Input: part model. Units: mm. Frame: model coordinates. A direction names the side the tool comes from. Coordinates: 2 decimals unless noted, no trailing zeros. Loops run counter-clockwise (first coordinate to the right, second up) from the corner with the lowest first, then second, coordinate; pieces in that order, holes last.
Item 1: Section A-A on z = 0. Return loops of the section in (x, y), and give its area (3 significant figures).
Item 2: Contact query for flat-ended pins moving along their axis: P1, Ø2, axis at x = -17, y = 4.5, coming from the +Z side; P2, Ø4.5, axis at x = -0.5, z = 0, coming from the +Y side; P3, Ø5.5, axis at x = -2, z = -1, coming from the -Y side. Output: stop coordinate, or through.
Item 3: Section B-B on x = -0.5. Return loops of the section in (y, z).
Item 4: Ray query, line 1 along Z through (x, y) = (-0.5, 10.45); line 2 along X through (y, z) = (-6, -22.5); line 3 along X through (y, z) = (5.5, 13). Return the intervals inside material, ascending.
Item 5: Reachability of faces 1 (the cylindrical face through (-2.25, 8.58, 0.08)), 2 (the flat face through (-1, 9.7, -2)), 3 (the cylindrical face through (1.08, -0.11, -3.05)) from +Z, -Z, +X, -X, +Y, -Y: full face, straight path, thin tool, end or side. Return the list, or none.
Item 6: Section C-C on y = 4. Return loops of the section in (x, z), and give its area (3 significant figures).
Item 7: Pull-direction query (X, two-part tool) for faces 4 (the cylindrical face through (4.344, 11.12, 1.525)), 5 (the flat face through (0, -7.5, -6)), 6 (the flat face through (2, 12.5, -2)); classes: released by +X, released by -X, zero draft, split by the parting line, or undercut.
```python
from build123d import *


with BuildPart() as part:
    # Esboço1 → Revolução1 (revolve)
    with BuildSketch(Plane.XY):
        with BuildLine():
            Line((30, -7.5), (30, -5.291502622))
            ThreePointArc((30, -5.291502622), (44, 0), (30, 5.291502622))
            Line((30, 5.291502622), (30, 7.5))
            Line((30, 7.5), (10, 7.5))
            Line((10, 7.5), (10, 9.7))
            Line((10, 9.7), (4.578419127, 9.7))
            Line((4.578419127, 9.7), (4.578419127, 12.5))
            Line((4.578419127, 12.5), (2.5, 12.5))
            Line((2.5, 12.5), (2.5, 9.7))
            Line((2.5, 9.7), (1.25, 9.7))
            Line((1.25, 9.7), (1.25, 7.5))
            Line((1.25, 7.5), (2.933342737, 7.5))
            Line((2.933342737, 7.5), (2.933342737, -7.5))
            Line((2.933342737, -7.5), (30, -7.5))
        make_face()
    revolve(axis=Axis((-0.5, 9.7, 0), (0, -1, 0)))


solid = part.part
```
Results found:
1. outline: (-31, -7.5) - (-3.93, -7.5) - (-3.93, 7.5) - (-2.25, 7.5) - (-2.25, 9.7) - (-3.5, 9.7) - (-3.5, 12.5) - (-5.58, 12.5) - (-5.58, 9.7) - (-11, 9.7) - (-11, 7.5) - (-31, 7.5) - (-31, 5.29) arc R8 ccw (long way) to (-31, -5.29) - close; (1.25, 7.5) - (2.93, 7.5) - (2.93, -7.5) - (30, -7.5) - (30, -5.29) arc R8 ccw (long way) to (30, 5.29) - (30, 7.5) - (10, 7.5) - (10, 9.7) - (4.58, 9.7) - (4.58, 12.5) - (2.5, 12.5) - (2.5, 9.7) - (1.25, 9.7) - close
1. area: 1,240 mm2
2. P1: stops at z = 40.59
2. P2: stops at y = 9.7
2. P3: stops at y = -7.5
3. outline: (-7.5, -30.5) - (-5.29, -30.5) arc R8 ccw (long way) to (5.29, -30.5) - (7.5, -30.5) - (7.5, -10.5) - (9.7, -10.5) - (9.7, -5.08) - (12.5, -5.08) - (12.5, -3) - (9.7, -3) - (9.7, -1.75) - (7.5, -1.75) - (7.5, -3.43) - (-7.5, -3.43) - close; (-7.5, 3.43) - (7.5, 3.43) - (7.5, 1.75) - (9.7, 1.75) - (9.7, 3) - (12.5, 3) - (12.5, 5.08) - (9.7, 5.08) - (9.7, 10.5) - (7.5, 10.5) - (7.5, 30.5) - (5.29, 30.5) arc R8 ccw (long way) to (-5.29, 30.5) - (-7.5, 30.5) - close
4. line 1: z = -5.08 to -3, 3 to 5.08
4. line 2: x = -35.72 to -22.13, -21.09 to 20.09, 21.13 to 34.72
4. line 3: x = -40.76 to -28.3, -28.09 to 27.09, 27.3 to 39.76
5. face 1: +Y, -Y
5. face 2: +Y
5. face 3: -Y
6. outline: circle Ø86.86 at (-0.5, 0); hole circle Ø6.87 at (-0.5, 0)
6. area: 5,890 mm2
7. face 4: split by the parting line
7. face 5: undercut
7. face 6: zero draft
